```python
from build123d import *

# Parameters (mm, degrees)
F0_R     = 177.8
F1_DEPTH = 4.7625
F3_D     = 10
F5_D     = 13
F7_D     = 17


with BuildPart() as f1:
    # F0 (on Front) → F1 (new body)
    with BuildSketch(Plane.XZ):
        Circle(F0_R)
    extrude(amount=F1_DEPTH)

    # F3 (through all)
    with Locations(Plane.XZ.offset(4.7625)):
        with Locations((0, 140), (53.575681, 129.343135), (98.994949, 98.994949), (129.343135, 53.575681), (140, 0), (129.343135, -53.575681), (98.994949, -98.994949), (53.575681, -129.343135), (0, -140), (-53.575681, -129.343135), (-98.994949, -98.994949), (-129.343135, -53.575681), (-140, 0), (-129.343135, 53.575681), (-98.994949, 98.994949), (-53.575681, 129.343135), (-53.575681, 129.343135)):
            Hole(F3_D / 2)

    # F5 (through all)
    with Locations(Plane.XZ.offset(4.7625)):
        with Locations((0, 80), (80, 0), (0, -80), (-80, 0)):
            Hole(F5_D / 2)

    # F7 (through all)
    with Locations(Plane.XZ.offset(4.7625)):
        with Locations((-70.710678, 70.710678)):
            Hole(F7_D / 2)


solid = f1.part
```
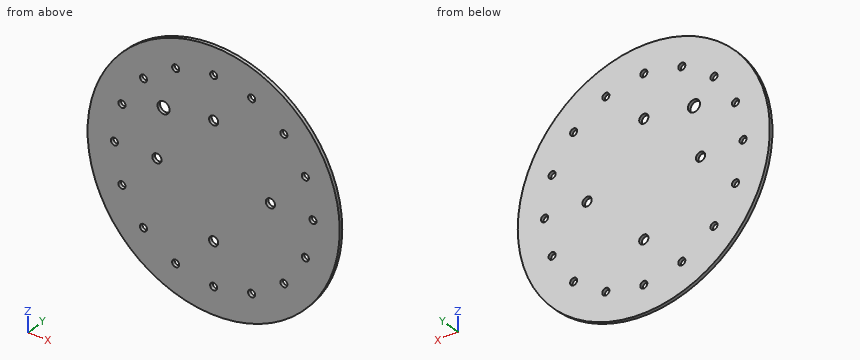
Here's how the part is built. I have some questions about the finished solid (model axes, mm). Coordinates: 2 decimals unless noted, no trailing zeros. Loops run counter-clockwise (first coordinate to the right, second up) from the corner with the lowest first, then second, coordinate; pieces in that order, holes last. Notation, with made-up numbers: (49, -15.75) -> (105, -15.75) arc R18 cw to (105, 14.25) -> close; hole circle Ø9 at (-18, 3). An arc over 180 degrees is marked (long way). Return JSON: item names as keys, results as strings.
1) If we section it at D-D, the plane z = 140: Write out the boundary of the cut face in (x, y).
Results below:
{"outline": "(-109.6, -4.76) -> (-5, -4.76) -> (-5, 0) -> (-109.6, 0) -> close; (5, -4.76) -> (109.6, -4.76) -> (109.6, 0) -> (5, 0) -> close"}
2) Will these pins go through, and if not, where does the flat tip stop? pin 1 (13 mm diameter, centred on x = -53.58, z = 129.34, fed in from +Y); pin 2 (1 mm diameter, centred on x = 93, y = -3, fed in from -Z).
Results below:
{"pin 1": "y = 0", "pin 2": "z = -151.84"}
3) I need wall thicknesses on line 1 (Z direction, x = 0, y = -2.6); line 2 (X direction, y = -1.3, z = -98); line 3 (X direction, y = -2.65, z = -102). Which ranges of each line are inside material? Lowest first, please. Write a range as from..to.
Results below:
{"line 1": "-177.8..-145, -135..-86.5, -73.5..73.5, 86.5..135, 145..177.8", "line 2": "-148.35..-103.89, -94.09..94.09, 103.89..148.35", "line 3": "-145.63..-102.99, -95..95, 102.99..145.63"}
4) If we section it at C-C, the plane y = -3.35: Count the separate pieces of the cut face and the enclosed holes in it, then the cut area to 3 significant figures.
Results below:
{"separate pieces": "1", "enclosed holes": "21", "area": "97,300 mm²"}
5) If we section it at A-A, the plane z = 0: Write out the boundary of the cut face in (x, y), then the cut area to 3 significant figures.
Results below:
{"outline": "(-177.8, -4.76) -> (-145, -4.76) -> (-145, 0) -> (-177.8, 0) -> close; (-135, -4.76) -> (-86.5, -4.76) -> (-86.5, 0) -> (-135, 0) -> close; (-73.5, -4.76) -> (73.5, -4.76) -> (73.5, 0) -> (-73.5, 0) -> close; (86.5, -4.76) -> (135, -4.76) -> (135, 0) -> (86.5, 0) -> close; (145, -4.76) -> (177.8, -4.76) -> (177.8, 0) -> (145, 0) -> close", "area": "1,470 mm²"}
6) If we section it at B-B, the plane x = 0: Write out the boundary of the cut face in (y, z), then the cut area to 3 significant figures.
Results below:
{"outline": "(-4.76, -177.8) -> (0, -177.8) -> (0, -145) -> (-4.76, -145) -> close; (-4.76, -135) -> (0, -135) -> (0, -86.5) -> (-4.76, -86.5) -> close; (-4.76, -73.5) -> (0, -73.5) -> (0, 73.5) -> (-4.76, 73.5) -> close; (-4.76, 86.5) -> (0, 86.5) -> (0, 135) -> (-4.76, 135) -> close; (-4.76, 145) -> (0, 145) -> (0, 177.8) -> (-4.76, 177.8) -> close", "area": "1,470 mm²"}
